from build123d import *

# Parameters (mm, degrees)
F0_R            = 38.1
F1_DEPTH        = 12.7
F3_DEPTH        = 12.7
F3_COPIES_COUNT = 15
F4_R            = 12.7
F5_DEPTH        = 101.6


# Not quite as in the source:
# - a pattern or mirror of a feature is missing from the dataset's text; its kind, count and spacing are read off the source's solid


with BuildPart() as f1:
    # F0 (on Front) → F1 (new body)
    with BuildSketch(Plane.XZ):
        Circle(F0_R)
    extrude(amount=F1_DEPTH)

    # F2 (on Front) → F3 (join, through all)
    with BuildSketch(Plane.XZ):
        Polygon((0, 50.8), (-7.798013599, 37.2934442484), (0, 38.1), align=None)
    f3 = extrude(amount=F3_DEPTH)

    # F3_copies: F3 ×15 about axis
    f3_copies_axis = Axis((0, 0, 0), (0, 1, 0))
    for i in range(1, F3_COPIES_COUNT):
        add(f3.rotate(f3_copies_axis, i * 360 / F3_COPIES_COUNT))

    # F4 (on Front) → F5 (join)
    with BuildSketch(Plane.XZ):
        Circle(F4_R)
    extrude(amount=F5_DEPTH)

    # F6 (on Right) → F7 (revolve, cut)
    with BuildSketch(Plane.YZ):
        with BuildLine():
            Line((-38.1, 17.78), (-65.8081287712, 17.78))
            ThreePointArc((-65.8081287712, 17.78), (-51.9540643856, 8.89), (-38.1, 17.78))
        make_face()
    revolve(axis=Axis((0, 0, 0), (0, 1, 0)), mode=Mode.SUBTRACT)


solid = f1.part
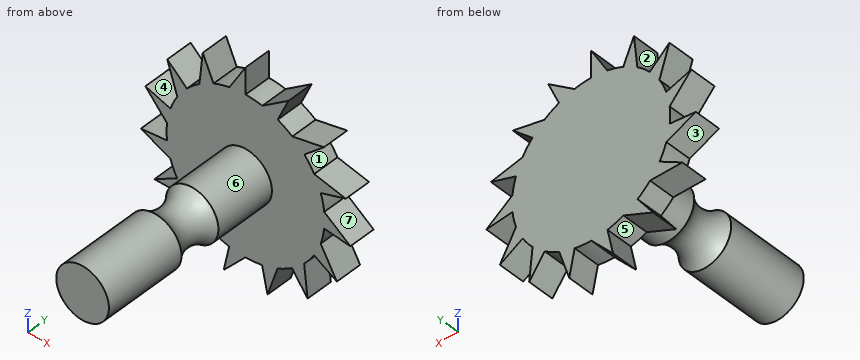
Here's how the part is built. I have some questions about the finished solid (model axes, mm). Face numbers are marked on the shaded views. A direction names the side the tool comes from. Round coordinates to 2 decimals unless told otherwise and drop trailing zeros. Loops run counter-clockwise (first coordinate to the right, second up) from the corner with the lowest first, then second, coordinate; pieces in that order, holes last.
1. If we section it at A-A on x = 41.5: Write out the boundary of the cut face in (y, z).
Answer list:
outline: (-12.7, -23.96) - (0, -23.96) - (0, -21.08) - (-12.7, -21.08) - close; (-12.7, -4.36) - (0, -4.36) - (0, 1.24) - (-12.7, 1.24) - close; (-12.7, 13.48) - (0, 13.48) - (0, 17.15) - (-12.7, 17.15) - close
2. If we section it at B-B on y = -89: Write out the boundary of the cut face in (x, z), plus the area to 3 significant figures.
Answer list:
outline: circle Ø25.4 at (0, 0)
area: 507 mm2
3. For P1, Ø12, axis at x = -3.5, y = -89.5, coming from the -Z side; P2, Ø3, axis at x = -0.5, z = 19.5, coming from the -Y side; P3, Ø8, axis at y = -31, z = 5.5, coming from the -X side, each with a flat end and sliding along its axis, tell me the tip position at first contact or that it passes through.
Answer list:
P1: stops at z = -12.7
P2: stops at y = -12.7
P3: stops at x = -12.61
4. If we section it at D-D on z = -15.5: Write out the boundary of the cut face in (x, y).
Answer list:
outline: (-34.8, -12.7) - (38.28, -12.7) - (38.28, 0) - (-34.8, 0) - close
5. If I drill on line 1 along X through (y, z) = (-3.5, 46); line 2 along Y through (x, z) = (-31, -1.5); line 3 along Y through (x, z) = (9.5, 7), over which ranges is the centre line in solid material (lowest first)?
Answer list:
line 1: x = -20.71 to -20.48, -2.77 to 0, 20.1 to 20.48
line 2: y = -12.7 to 0
line 3: y = -101.6 to -60.91, -43 to 0
6. We'd pull the mould along X, two halves only. Please class the marked faces 1, 2, 3 and 4: +X half, -X half, draft (parallel to the pull), parting line (faces both ways), or undercut.
Answer list:
face 1: +X half
face 2: undercut
face 3: -X half
face 4: undercut
7. Which directions (+Z, -Z, +X, -X, +Y, -Y) give clear straight access to the entire face, cutting with the end or side of a thin tool? Please do the marked faces 5, 6 and 7.
Answer list:
face 5: +Y, -Y
face 6: -Y
face 7: +X, +Y, -Y
8. If we section it at C-C on z = 0: Write out the boundary of the cut face in (x, y), plus the area to 3 significant figures.
Answer list:
outline: (-38.1, -12.7) - (-12.7, -12.7) - (-12.7, -41.87) arc R15.24 cw to (-12.7, -62.03) - (-12.7, -101.6) - (12.7, -101.6) - (12.7, -62.03) arc R15.24 cw to (12.7, -41.87) - (12.7, -12.7) - (43.21, -12.7) - (43.21, 0) - (-38.1, 0) - close
area: 3,190 mm2
